For this review, take the finished solid that the model builds, in its own axes (mm). A direction names the side the tool comes from. Coordinates: 2 decimals unless noted, no trailing zeros. Order: outer loops, then holes, each group sorted by start corner. A loop starts at its lowest first (then second) coordinate and runs counter-clockwise, first axis right, second up.
from build123d import *

# Parameters (mm, degrees)
SKETCH3_W                    = 131
SKETCH3_H                    = 54
BOSS_EXTRUDE2_DEPTH          = 5
F_3_0_3_DIAMETER_HOLE1_D     = 3
F_3_0_3_DIAMETER_HOLE1_DEPTH = 20
F_3_0_3_DIAMETER_HOLE1_TIP   = 0.901290929
SHELL1_T                     = -1.5
CUT_EXTRUDE1_DEPTH           = 114.452633288
FILLET2_START                = -28
FILLET2_DEPTH                = 120.497573337
FILLET2_2_ANGLE              = 180


with BuildPart() as part:
    # Sketch3 → Boss-Extrude2 (new body)
    with BuildSketch(Plane.XY):
        with BuildLine():
            Line((-65.5, 27), (65.5, 27))
            ThreePointArc((65.5, 27), (0, 92.5), (-65.5, 27))
        make_face()
        Rectangle(SKETCH3_W, SKETCH3_H)
    extrude(amount=BOSS_EXTRUDE2_DEPTH)

    # Ø3.0 (3) Diameter Hole1
    with Locations(Plane.XY.offset(5)):
        with Locations((-63.5, -17), (63.5, -17), (0, 89.5), (63.5, 31.210132452), (-63.5, 31.210132452)):
            Hole(F_3_0_3_DIAMETER_HOLE1_D / 2, depth=F_3_0_3_DIAMETER_HOLE1_DEPTH)
            with Locations((0, 0, -(F_3_0_3_DIAMETER_HOLE1_DEPTH + F_3_0_3_DIAMETER_HOLE1_TIP / 2))):  # 118° drill point
                Cone(0, F_3_0_3_DIAMETER_HOLE1_D / 2, F_3_0_3_DIAMETER_HOLE1_TIP, mode=Mode.SUBTRACT)

    # Shell1
    shell1_openings = [part.faces().sort_by_distance(p)[0] for p in [
        (0, 26.743328941, 5),
    ]]
    offset(amount=SHELL1_T, openings=shell1_openings)

    # Sketch6 → Cut-Extrude1 (cut, through all)
    with BuildSketch(Plane(origin=(0, 0, 0), x_dir=(-1, 0, 0), z_dir=(0, 0, -1))):
        with BuildLine():
            Line((-6, 27), (-6, -27))
            Line((-6, -27), (6, -27))
            Line((6, -27), (6, 27))
            ThreePointArc((6, 27), (0, 33), (-6, 27))
        make_face()
    extrude(amount=-CUT_EXTRUDE1_DEPTH, mode=Mode.SUBTRACT)

    # Fillet2: read off the stored shape, not the designer's step
    # Fillet2 outline → Fillet2 (cut)
    with BuildSketch(Plane(origin=(0, 0, 0), x_dir=(1, 0, 0), z_dir=(0, 1, 0)).offset(FILLET2_START)):
        with BuildLine():
            ThreePointArc((-65.5, -2.5), (-64.767766953, -0.732233047), (-63, 0))
            Line((-63, 0), (-65.5, 0))
            Line((-65.5, 0), (-65.5, -2.5))
        make_face()
        with BuildLine():
            ThreePointArc((63, 0), (64.767766953, -0.732233047), (65.5, -2.5))
            Line((65.5, -2.5), (65.5, 0))
            Line((65.5, 0), (63, 0))
        make_face()
    extrude(amount=FILLET2_DEPTH, mode=Mode.SUBTRACT)

    # Fillet2 2 outline → Fillet2 2 (revolve, cut)
    with BuildSketch(Plane.XZ.offset(-27)):
        with BuildLine():
            ThreePointArc((65.5, 2.5), (64.767766953, 0.732233047), (63, 0))
            Line((63, 0), (65.5, 0))
            Line((65.5, 0), (65.5, 2.5))
        make_face()
    revolve(axis=Axis((0, 27, 0), (0, 0, 1)), revolution_arc=FILLET2_2_ANGLE, mode=Mode.SUBTRACT)


solid = part.part
1. Machinability: for faces 5 (the face through (-64, -23, 3)), 6 (the face through (35, -27, 2)), 7 (the face through (6, -2, 1)), which of the approach directions +Z, -Z, +X, -X, +Y, -Y give a long, thin tool a straight path to every point of the face, cutting with its end or side? Answer none if there is none.
Answer below:
face 5: +Z
face 6: +Z, -Z, +X, -X, -Y
face 7: +Z, -Z, -Y
2. Clearance check with flat-ended pins moving along their axes: pin 1 Ø1.8 at (x, z) = (30.5, 2.5) entering from +Y; pin 2 Ø1.5 at (x, z) = (46, 2.5) entering from +Y; pin 3 Ø1.5 at (y, z) = (32, 3.5) entering from +X. State where each tip first meets the part, or that it passes through.
Answer below:
pin 1: stops at y = 85.43
pin 2: stops at y = 74.36
pin 3: stops at x = 65.36
3. Take a section at A-A, the plane x = 0. Give the boundary of the cut face in (y, z).
Answer below:
outline: (33, 0) - (88, 0) - (88, 5) - (86.5, 5) - (86.5, 1.5) - (33, 1.5) - close; (91, 0.21) arc R2.5 ccw to (92.5, 2.5) - (92.5, 5) - (91, 5) - close
4. To check wall thickness, follow L1, parallel to Z at x = -35, y = 26; L2, parallel to X at y = 1, z = 3.85; L3, parallel to Y at x = -40, z = 4.3. State the ranges of each line that lie inside material, in increasing order.
Answer below:
L1: z = 0 to 1.5
L2: x = -65.5 to -64, 64 to 65.5
L3: y = -27 to -25.5, 76.96 to 78.87
5. The part is to be moulded in two halves that separate along Y. For faces 1 (the face through (-60.5, -16.9, 3.2)), 2 (the face through (-6, -2, 1)), 3 (the face through (-36, -27, 2)), 4 (the face through (-62, 31.28, 2.46)), say which applies: +Y half, -Y half, draft (parallel to the pull), parting line (faces both ways), or undercut.
Answer below:
face 1: undercut
face 2: draft
face 3: -Y half
face 4: undercut
